Geometry: final body of the model. Coordinates: model frame, mm. A direction names the side the tool comes from. Coordinates: 2 decimals unless noted, no trailing zeros. Order: outer loops, then holes, each group sorted by start corner. A loop starts at its lowest first (then second) coordinate and runs counter-clockwise, first axis right, second up. Notation, with made-up numbers: (38.25, -39.75) -> (45.25, -39.75) arc R13 cw to (45.25, -14.75) -> close; hole circle Ø6 at (18.5, -2). An arc over 180 degrees is marked (long way). Answer in a Markdown table with one row per item. Add a question column.
1) Contact query for flat-ended pins moving along their axis: P1, Ø10, axis at x = -94, z = 34.5, coming from the +Y side; P2, Ø10, axis at y = -58, z = -43, coming from the +X side; P3, Ø10, axis at x = 4, y = -31.5, coming from the +Z side; P4, Ø15, axis at x = -88.9, z = 31.75, coming from the +Y side. Output: stop coordinate, or through.
2) Section query D-D on x = -110. Return the cut outline in (y, z), then the cut area to 3 significant figures.
3) Pull-direction query (Z, two-part tool) for faces 1 (the face through (-84.5, -63.7, -40.2)), 2 (the face through (-43.56, -63.68, 20.34)), 3 (the face through (-80, -64, -50.8)), 4 (the face through (24.44, 29.23, -0.18)); classes: +Z half, -Z half, draft (parallel to the pull), parting line (faces both ways), or undercut.
4) Set-up query: faces 5 (the face through (-77, -50.8, 32)), 6 (the face through (-77, -50.8, -31)), 7 (the face through (-50.8, -64, -45)), 8 (the face through (-121.57, -63.68, -45.07)), 9 (the face through (-121.27, -63.68, 45.37)). Return all of +Z, -Z, +X, -X, +Y, -Y with unobstructed straight access to the full face (end or side cutting, diameter ignored); none if empty.
5) Ray query, line 1 (Z direction, x = -88.9, y = -70.5) (3 decimals); line 2 (Z direction, x = -88, y = -61); line 3 (Y direction, x = 0, z = -7) (3 decimals). Return the intervals inside material, ascending. Write a range as from..to.
6) Section query C-C on x = -88.9. Return the cut outline in (y, z) (3 decimals), then the cut area to 3 significant figures.
7) Section query A-A on y = 0. Return the cut outline in (x, z) (3 decimals).
8) Section query B-B on z = -27.5. Return the cut outline in (x, y), then the cut area to 3 significant figures.
Autodesk Inventor part; units mm, degrees
ref_plane "YZ Plane" through (0, 0, 0) normal (1, 0, 0) x (0, 1, 0)
ref_plane "XZ Plane" through (0, 0, 0) normal (0, 1, 0) x (-1, 0, 0)
ref_plane "XY Plane" through (0, 0, 0) normal (0, 0, 1) x (1, 0, 0)
sketch "Sketch1" plane through (0, 0, 0) normal (0, 0, 1) x (1, 0, 0)
  circle A0 centre (0, 0) radius 22.225
  arc A1 (32.9956, -19.05) -> (-23.4434, 30.0336) centre (0, 0) ccw
  line L0 (32.9956, -19.05) -> (0, -76.2)
  line L1 (0, -76.2) -> (-127, -76.2)
  line L2 (-127, -76.2) -> (-127, -50.8)
  line L3 (-127, -50.8) -> (-23.4434, 30.0336)
  dimension "d0" = 44.45
  dimension "d1" = 38.1
  dimension "d2" = 76.2
  dimension "d3" = 127
  dimension "d4" = 25.4
extrude "Extrusion1" add sketch "Sketch1" along normal mid plane 25.4
sketch "Sketch2" plane through (-127, -76.2, 12.7) normal (0, -1, 0) x (1, 0, 0)
  line L0 (0, -25.4) -> (0, 0) construction
  line L1 (0, -12.7) -> (165.1, -12.7) construction
  line L2 (165.1, -25.4) -> (165.1, 0) construction
  line L3 (0, -12.7) -> (0, 19.05)
  line L4 (19.05, 38.1) -> (76.2, 38.1)
  line L5 (76.2, 38.1) -> (76.2, 25.4)
  line L6 (76.2, 25.4) -> (76.2, 0.0039) construction
  arc A0 (76.2, 25.4) -> (101.6, 0) centre (101.6, 25.4) ccw
  line L7 (101.6, 0) -> (0, 0)
  circle A1 centre (38.1, 19.05) radius 9.525
  arc A2 (19.05, 38.1) -> (0, 19.05) centre (19.05, 19.05) ccw
  line L8 (0, 0) -> (0, -25.4) construction
  line L9 (0, -12.7) -> (0, -44.45)
  line L10 (19.05, -63.5) -> (76.2, -63.5)
  line L11 (76.2, -63.5) -> (76.2, -50.8)
  line L12 (76.2, -50.8) -> (76.2, -25.4039) construction
  arc A3 (101.6, -25.4) -> (76.2, -50.8) centre (101.6, -50.8) ccw
  line L13 (101.6, -25.4) -> (0, -25.4)
  circle A4 centre (38.1, -44.45) radius 9.525
  arc A5 (0, -44.45) -> (19.05, -63.5) centre (19.05, -44.45) ccw
  point P0 (127, -12.7)
  point P1 (0, 38.1)
  point P2 (0, -63.5)
  dimension "d7" = 19.05
  dimension "d8" = 101.6
  dimension "d9" = 19.05
  dimension "d10" = 76.2
  dimension "d11" = 25.4
  dimension "d12" = 19.05
  dimension "d13" = 38.1
extrude "Extrusion2" add sketch "Sketch2" against normal blind 25.4
properties part number "AnchorBase"
Result:
| question | item | result |
|---|---|---|
| 1 | P1 | y = -50.8 |
| 1 | P2 | x = -50.8 |
| 1 | P3 | z = 12.7 |
| 1 | P4 | through |
| 2 | outline | (-76.2, -50.69) -> (-50.8, -50.69) -> (-50.8, -12.7) -> (-37.53, -12.7) -> (-37.53, 12.7) -> (-50.8, 12.7) -> (-50.8, 50.69) -> (-76.2, 50.69) -> close |
| 2 | area | 2,910 mm2 |
| 3 | face 1 | undercut |
| 3 | face 2 | +Z half |
| 3 | face 3 | -Z half |
| 3 | face 4 | draft |
| 4 | face 5 | +Z, +X, -X, +Y |
| 4 | face 6 | -Z, +X, -X, +Y |
| 4 | face 7 | -Z, +X, +Y, -Y |
| 4 | face 8 | -Z, -X, +Y, -Y |
| 4 | face 9 | +Z, -X, +Y, -Y |
| 5 | line 1 | -50.8..-41.275, -22.225..22.225, 41.275..50.8 |
| 5 | line 2 | -50.8..-41.23, -22.27..22.27, 41.23..50.8 |
| 5 | line 3 | -76.2..-22.225, 22.225..38.1 |
| 6 | outline | (-76.2, -50.8) -> (-50.8, -50.8) -> (-50.8, -41.275) -> (-76.2, -41.275) -> close; (-76.2, -22.225) -> (-50.8, -22.225) -> (-50.8, -12.7) -> (-21.06, -12.7) -> (-21.06, 12.7) -> (-50.8, 12.7) -> (-50.8, 22.225) -> (-76.2, 22.225) -> close; (-76.2, 41.275) -> (-50.8, 41.275) -> (-50.8, 50.8) -> (-76.2, 50.8) -> close |
| 6 | area | 2,370 mm2 |
| 7 | outline | (-61.92, -12.7) -> (-22.225, -12.7) -> (-22.225, 12.7) -> (-61.92, 12.7) -> close; (22.225, -12.7) -> (38.1, -12.7) -> (38.1, 12.7) -> (22.225, 12.7) -> close |
| 8 | outline | (-127, -76.2) -> (-97.42, -76.2) -> (-97.42, -50.8) -> (-127, -50.8) -> close; (-80.38, -76.2) -> (-48.48, -76.2) -> (-48.48, -50.8) -> (-80.38, -50.8) -> close |
| 8 | area | 1,560 mm2 |
